from build123d import *

# Parameters (mm, degrees)
F1_DEPTH       = 2
F3_D           = 8.8
F3_CSINK_D     = 17.92
F3_CSINK_ANGLE = 90


with BuildPart() as f1:
    # F0 (on Top) → F1 (new body)
    with BuildSketch(Plane.XY):
        Polygon((-81.1824680357, 67), (-42.5, 0), (42.5, 0), (81.1824680357, 67), align=None)
    extrude(amount=F1_DEPTH)

    # F3 (through all)
    with Locations(Plane.XY.offset(2)):
        with Locations((0, 47)):
            CounterSinkHole(F3_D / 2, F3_CSINK_D / 2, counter_sink_angle=F3_CSINK_ANGLE)


solid = f1.part
Can you work these out from the model? Positions are in its coordinate system, mm. Give positions to 0.01 mm unless a question says otherwise; leave off trailing zeros. Loops run counter-clockwise (first coordinate to the right, second up) from the corner with the lowest first, then second, coordinate; pieces in that order, holes last. Notation, with made-up numbers: (7.25, 41) - (64.25, 41) arc R10 cw to (64.25, 53) - close; hole circle Ø2 at (-37, 48.25). An arc over 180 degrees is marked (long way). Return JSON: item names as keys, results as strings.
1. I want a section at B-B on z = 1.5. Please give me the cut outline in (x, y), and give its area (3 significant figures).
Output values:
{"outline": "(-81.18, 67) - (-42.5, 0) - (42.5, 0) - (81.18, 67) - close; hole circle Ø16.92 at (0, 47)", "area": "8,060 mm²"}
2. I'm going to push a flat-ended pin straight in: pin 1 Ø1 at (y, z) = (49, 1) entering from -X. Where does the tip first touch, or does it pass through?
Output values:
{"pin 1": "stops at x = -71.08"}
3. I want a section at A-A on x = 0. Please give me the cut outline in (y, z).
Output values:
{"outline": "(0, 0) - (40.04, 0) - (38.04, 2) - (0, 2) - close; (53.96, 0) - (67, 0) - (67, 2) - (55.96, 2) - close"}
4. If I drill on line 1 (X direction, y = 41, z = 0.1); line 2 (X direction, y = 48, z = 1.05); line 3 (Y direction, x = 43, z = 0.8), over which ranges is the centre line in solid material (lowest first)?
Output values:
{"line 1": "x = -66.17 to -3.72, 3.72 to 66.17", "line 2": "x = -70.21 to -7.95, 7.95 to 70.21", "line 3": "y = 0.87 to 67"}
5. I want a section at C-C on y = 47. Please give me the cut outline in (x, z).
Output values:
{"outline": "(-69.64, 0) - (-6.96, 0) - (-8.96, 2) - (-69.64, 2) - close; (6.96, 0) - (69.64, 0) - (69.64, 2) - (8.96, 2) - close"}
6. I want a section at D-D on y = 21. Please give me the cut outline in (x, z), and give its area (3 significant figures).
Output values:
{"outline": "(-54.62, 0) - (54.62, 0) - (54.62, 2) - (-54.62, 2) - close", "area": "218 mm²"}
